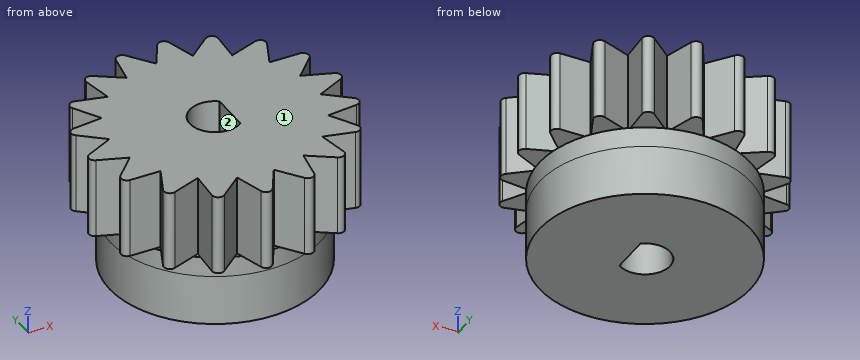
```python
from build123d import *

# Parameters (mm, degrees)
SKETCH1_R                 = 7.5
BOSS_EXTRUDE1_DEPTH       = 10
SKETCH3_R                 = 10.5
BOSS_EXTRUDE2_DEPTH       = 5
CUT_EXTRUDE1_REACH        = 23.107
BOSS_EXTRUDE3_START       = -8
SKETCH4_R                 = 14.5
SKETCH4_R_2               = 7.5
BOSS_EXTRUDE3_DEPTH       = 8
BOSS_EXTRUDE4_OUTLINE_R   = 10.5
BOSS_EXTRUDE4_OUTLINE_R_2 = 7.5
BOSS_EXTRUDE4_DEPTH       = 2
SKETCH6_R                 = 14.465552515
CUT_EXTRUDE2_DEPTH        = 8


# Read off the part's stored shape, not the designer's step: Boss-Extrude4
with BuildPart() as part:
    # Sketch1 → Boss-Extrude1 (new body)
    with BuildSketch(Plane.XY):
        Circle(SKETCH1_R)
    extrude(amount=BOSS_EXTRUDE1_DEPTH)

    # Sketch3 → Boss-Extrude2 (add)
    with BuildSketch(Plane(origin=(0, 0, 0), x_dir=(-1, 0, 0), z_dir=(0, 0, -1))):
        Circle(SKETCH3_R)
    extrude(amount=BOSS_EXTRUDE2_DEPTH)

    # Sketch2 → Cut-Extrude1 (cut, up to next)
    with BuildSketch(Plane.XY.offset(10), mode=Mode.PRIVATE) as cut_extrude1_sk1:
        with BuildLine():
            Line((1.5, 2), (1.5, -2))
            ThreePointArc((1.5, -2), (-2.5, 0), (1.5, 2))
        make_face()
    cut_extrude1_tool1 = extrude(cut_extrude1_sk1.sketch, amount=-CUT_EXTRUDE1_REACH, mode=Mode.PRIVATE) & part.part
    add(cut_extrude1_tool1.solids().sort_by_distance((-0.316718, 0, 10))[0], mode=Mode.SUBTRACT)

    # Sketch4 → Boss-Extrude3 (add)
    with BuildSketch(Plane.XY.offset(10).offset(BOSS_EXTRUDE3_START)):
        Circle(SKETCH4_R)
        with Locations(Location((0, 0, 0), (0, 0, 180))):
            Circle(SKETCH4_R_2, mode=Mode.SUBTRACT)
    extrude(amount=BOSS_EXTRUDE3_DEPTH)

    # Boss-Extrude4 outline → Boss-Extrude4 (add)
    with BuildSketch(Plane.XY):
        Circle(BOSS_EXTRUDE4_OUTLINE_R)
        Circle(BOSS_EXTRUDE4_OUTLINE_R_2, mode=Mode.SUBTRACT)
    extrude(amount=BOSS_EXTRUDE4_DEPTH)

    # Sketch6 → Cut-Extrude2 (cut)
    with BuildSketch(Plane.XY.offset(10)):
        Circle(SKETCH6_R)
        with BuildLine():
            Line((5.915587052, 8.062619291), (6.088339002, 11.088366247))
            ThreePointArc((6.088339002, 11.088366247), (5.754853945, 11.660608595), (5.097799094, 11.57722688))
            Line((5.097799094, 11.57722688), (2.801255295, 9.599633783))
            Line((2.801255295, 9.599633783), (1.92872262, 12.501990517))
            ThreePointArc((1.92872262, 12.501990517), (1.419630763, 12.925663822), (0.830719394, 12.622584645))
            Line((0.830719394, 12.622584645), (-0.650949193, 9.978790766))
            Line((-0.650949193, 9.978790766), (-2.463526175, 12.407690221))
            ThreePointArc((-2.463526175, 12.407690221), (-3.086820841, 12.631693229), (-3.536557325, 12.145472413))
            Line((-3.536557325, 12.145472413), (-4.024639601, 9.154358311))
            Line((-4.024639601, 9.154358311), (-6.558637356, 10.816839366))
            ThreePointArc((-6.558637356, 10.816839366), (-7.220956294, 10.814154009), (-7.477273036, 10.203436959))
            Line((-7.477273036, 10.203436959), (-6.912899076, 7.225775139))
            Line((-6.912899076, 7.225775139), (-9.862680076, 7.921318044))
            ThreePointArc((-9.862680076, 7.921318044), (-10.484137849, 7.692268216), (-10.516119267, 7.030716422))
            Line((-10.516119267, 7.030716422), (-8.967360899, 4.425656845))
            Line((-8.967360899, 4.425656845), (-11.977138021, 4.07036886))
            ThreePointArc((-11.977138021, 4.07036886), (-12.48277765, 3.64258135), (-12.286566313, 3.009987721))
            Line((-12.286566313, 3.009987721), (-9.940226653, 1.09173902))
            Line((-9.940226653, 1.09173902), (-12.646976358, -0.271526881))
            ThreePointArc((-12.646976358, -0.271526881), (-12.97581024, -0.846454586), (-12.575072131, -1.373789921))
            Line((-12.575072131, -1.373789921), (-9.714154371, -2.373858644))
            Line((-9.714154371, -2.373858644), (-11.791402696, -4.580672473))
            ThreePointArc((-11.791402696, -4.580672473), (-11.903768612, -5.233395606), (-11.346838661, -5.591868224))
            Line((-11.346838661, -5.591868224), (-8.316411706, -5.553133921))
            Line((-8.316411706, -5.553133921), (-9.513611846, -8.337321361))
            ThreePointArc((-9.513611846, -8.337321361), (-9.395956809, -8.98911188), (-8.750008988, -9.135484692))
            Line((-8.750008988, -9.135484692), (-5.915587052, -8.062619291))
            Line((-5.915587052, -8.062619291), (-6.088339002, -11.088366247))
            ThreePointArc((-6.088339002, -11.088366247), (-5.754853945, -11.660608595), (-5.097799094, -11.57722688))
            Line((-5.097799094, -11.57722688), (-2.801255295, -9.599633783))
            Line((-2.801255295, -9.599633783), (-1.92872262, -12.501990517))
            ThreePointArc((-1.92872262, -12.501990517), (-1.419630763, -12.925663822), (-0.830719394, -12.622584645))
            Line((-0.830719394, -12.622584645), (0.650949193, -9.978790766))
            Line((0.650949193, -9.978790766), (2.463526175, -12.407690221))
            ThreePointArc((2.463526175, -12.407690221), (3.086820841, -12.631693229), (3.536557325, -12.145472413))
            Line((3.536557325, -12.145472413), (4.024639601, -9.154358311))
            Line((4.024639601, -9.154358311), (6.558637356, -10.816839366))
            ThreePointArc((6.558637356, -10.816839366), (7.220956294, -10.814154009), (7.477273036, -10.203436959))
            Line((7.477273036, -10.203436959), (6.912899076, -7.225775139))
            Line((6.912899076, -7.225775139), (9.862680076, -7.921318044))
            ThreePointArc((9.862680076, -7.921318044), (10.484137849, -7.692268216), (10.516119267, -7.030716422))
            Line((10.516119267, -7.030716422), (8.967360899, -4.425656845))
            Line((8.967360899, -4.425656845), (11.977138021, -4.07036886))
            ThreePointArc((11.977138021, -4.07036886), (12.48277765, -3.64258135), (12.286566313, -3.009987721))
            Line((12.286566313, -3.009987721), (9.940226653, -1.09173902))
            Line((9.940226653, -1.09173902), (12.646976358, 0.271526881))
            ThreePointArc((12.646976358, 0.271526881), (12.97581024, 0.846454586), (12.575072131, 1.373789921))
            Line((12.575072131, 1.373789921), (9.714154371, 2.373858644))
            Line((9.714154371, 2.373858644), (11.791402696, 4.580672473))
            ThreePointArc((11.791402696, 4.580672473), (11.903768612, 5.233395606), (11.346838661, 5.591868224))
            Line((11.346838661, 5.591868224), (8.316411706, 5.553133921))
            Line((8.316411706, 5.553133921), (9.513611846, 8.337321361))
            ThreePointArc((9.513611846, 8.337321361), (9.395956809, 8.98911188), (8.750008988, 9.135484692))
            Line((8.750008988, 9.135484692), (5.915587052, 8.062619291))
        make_face(mode=Mode.SUBTRACT)
    extrude(amount=-CUT_EXTRUDE2_DEPTH, mode=Mode.SUBTRACT)


with BuildPart() as body_2:
    # of the pieces the cut leaves, the one that is kept (cut_extrude2_keep)
    add(part.part.solids().sort_by_distance((-10.5, 0, 0))[0])


solid = body_2.part
```
Could you check a few things on this model? Use its own coordinates, in mm. Face numbers are marked on the shaded views. A direction names the side the tool comes from. Round coordinates to 2 decimals unless told otherwise and drop trailing zeros. Write each loop counter-clockwise with the first axis right and the second up, starting at its lowest first coordinate (ties: lowest second). Pieces come first, ordered by that corner, then holes.
(1) For pin 1 (1 mm diameter, centred on y = 9.5, z = 8, fed in from -X); pin 2 (0.9 mm diameter, centred on x = 2, y = -11, fed in from -Z); pin 3 (1.5 mm diameter, centred on y = 7.5, z = 4.5, fed in from +X), each with a flat end and sliding along its axis, tell me the tip position at first contact or that it passes through.
Findings below:
pin 1: stops at x = -7.44
pin 2: stops at z = 2
pin 3: stops at x = 9.48
(2) Suppose I cut it at C-C on y = 3.5. Write out the boundary of the cut face in (x, z).
Findings below:
outline: (-12.51, 2) - (-9.9, 2) - (-9.9, -5) - (9.9, -5) - (9.9, 2) - (10.77, 2) - (10.77, 10) - (-12.51, 10) - close
(3) Suppose I cut it at B-B on z = 1.5. Write out the boundary of the cut face in (x, y), and give its area (3 significant figures).
Findings below:
outline: circle Ø21 at (0, 0); hole (1.5, -2) - (1.5, 2) arc R2.5 ccw (long way) to start
area: 330 mm2
(4) If I drill on probe 1 along Y at (x, z) = (11, 7.75); probe 2 along X at (y, z) = (0, -1); probe 3 along X at (y, z) = (0, 6.75), over which ranges is the centre line in solid material (lowest first)?
Findings below:
probe 1: y = -4.19 to -1.96, -0.56 to 1.92, 3.74 to 5.59
probe 2: x = -10.5 to -2.5, 1.5 to 10.5
probe 3: x = -12.11 to -2.5, 1.5 to 12.11
(5) Suppose I cut it at A-A on x = 0. Write out the boundary of the cut face in (y, z).
Findings below:
outline: (-11.14, 2) - (-10.5, 2) - (-10.5, -5) - (-2.5, -5) - (-2.5, 10) - (-11.14, 10) - close; (2.5, -5) - (10.5, -5) - (10.5, 2) - (11.14, 2) - (11.14, 10) - (2.5, 10) - close
(6) Which directions (+Z, -Z, +X, -X, +Y, -Y) give clear straight access to the entire face, cutting with the end or side of a thin tool? Please do the marked faces 1 and 2.
Findings below:
face 1: +Z, +X, -X, +Y, -Y
face 2: +Z, -Z
